```python
from build123d import *

# Parameters (mm, degrees)
F0_R     = 17.65
F1_DEPTH = 33
F2_R     = 2.65
F3_DEPTH = 3.5
F5_DEPTH = 3.5


with BuildPart() as f1:
    # F0 (on Top) → F1 (new body)
    with BuildSketch(Plane.XY):
        Circle(F0_R)
    extrude(amount=F1_DEPTH)

    # F2 (on face) → F3 (join)
    with BuildSketch(Plane.XY.offset(33)):
        Circle(F2_R)
    extrude(amount=F3_DEPTH)

    # F4 (on face) → F5 (join)
    with BuildSketch(Plane.XY.offset(33)):
        with BuildLine():
            ThreePointArc((0.2, -2.6424420523), (0, -2.65), (-0.2, -2.6424420523))
            Line((-0.2, -2.6424420523), (-0.2, -3.0434355587))
            Line((-0.2, -3.0434355587), (0, -3.0434355587))
            Line((0, -3.0434355587), (0.2, -3.0434355587))
            Line((0.2, -3.0434355587), (0.2, -2.6424420523))
        make_face()
    extrude(amount=F5_DEPTH)


solid = f1.part
```
Verification items for the finished model (mm, model axes). A direction names the side the tool comes from. Coordinates: 2 decimals unless noted, no trailing zeros. Write each loop counter-clockwise with the first axis right and the second up, starting at its lowest first coordinate (ties: lowest second). Pieces come first, ordered by that corner, then holes. Notation, with made-up numbers: (28.5, -11) - (50.5, -11) arc R27 ccw to (50.5, 22) - close; hole circle Ø5 at (64, -32.75). An arc over 180 degrees is marked (long way). Write item = value, one per line.
Q1. Cross-section at B-B (z = 21.5). Enter the section's corners in (x, y).
Answer:
outline = circle Ø35.3 at (0, 0)
Q2. Material ranges on L1, parallel to Z at x = 5.5, y = -3; L2, parallel to Y at x = -12, z = 27; L3, parallel to X at y = 6, z = 14, recorded low to high. Write a range as from..to.
Answer:
L1 = 0..33
L2 = -12.94..12.94
L3 = -16.6..16.6
Q3. Cross-section at C-C (x = -1). Enter the section's corners in (y, z), plus the area to 3 significant figures.
Answer:
outline = (-17.62, 0) - (17.62, 0) - (17.62, 33) - (2.45, 33) - (2.45, 36.5) - (-2.45, 36.5) - (-2.45, 33) - (-17.62, 33) - close
area = 1,180 mm²
Q4. Cross-section at D-D (y = 10). Enter the section's corners in (x, z).
Answer:
outline = (-14.54, 0) - (14.54, 0) - (14.54, 33) - (-14.54, 33) - close
Q5. Go/stop test with flat-tipped pins: pin 1 Ø1.5 at (x, z) = (-6.5, 13) entering from +Y; pin 2 Ø1.5 at (x, z) = (12.5, 28.5) entering from +Y; pin 3 Ø1.5 at (x, z) = (-10, 10.5) entering from -Y. Record where each tip stops, or that it passes through.
Answer:
pin_1 = 16.69
pin_2 = 13.17
pin_3 = -15.03
Q6. Access from +Z, -Z, +X, -X, +Y, -Y to the whole of each face (thin tool, end or side, straight path). Record for faces 1 (the face through (0, 0, 0)), 2 (the face through (0.114, 2.648, 34.726)).
Answer:
face_1 = -Z, +X, -X, +Y, -Y
face_2 = +Z
Q7. Cross-section at A-A (y = 0). Enter the section's corners in (x, z).
Answer:
outline = (-17.65, 0) - (17.65, 0) - (17.65, 33) - (2.65, 33) - (2.65, 36.5) - (-2.65, 36.5) - (-2.65, 33) - (-17.65, 33) - close
